Autodesk Inventor part; units mm, degrees
ref_plane "YZ Plane" through (0, 0, 0) normal (1, 0, 0) x (0, 1, 0)
ref_plane "XZ Plane" through (0, 0, 0) normal (0, 1, 0) x (-1, 0, 0)
ref_plane "XY Plane" through (0, 0, 0) normal (0, 0, 1) x (1, 0, 0)
sketch "Sketch1" plane through (0, 0, 0) normal (1, 0, 0) x (0, 1, 0)
  line L0 (-32.2, 0) -> (32.2, 0)
  line L1 (0, -4.2) -> (0, 4.2)
  circle A0 centre (-20, 0) radius 1.25
  circle A1 centre (-20, 0) radius 3
  circle A2 centre (20, 0) radius 3 construction
  line L2 (-20, 3) -> (20, 3)
  line L3 (-20, -3) -> (20, -3)
  line L4 (20, 3) -> (20, -3) construction
  line L5 (20, 2) -> (20, -2) construction
  arc A3 (20, -3) -> (20, 3) centre (20, 0) ccw
  circle A4 centre (-20, 0) radius 2.2678 construction
  circle A5 centre (20, 0) radius 1
  point P0 (0, 0)
  dimension "d4" = 6
  dimension "d7" = 40
  dimension "d8" = 2.5
  dimension "d10" = 0
  dimension "d30" = 2
extrude "ext_main" add sketch "Sketch1" along normal mid plane 3.5 contours A0 L0 A1 | L0 A1 A0 | A1 L2 L1 L0 | L0 L1 L3 A1 | L1 L2 A3 L0 A5 | L0 A5 A3 L3 L1
sketch "Sketch3" plane through (0, 0, 0) normal (1, 0, 0) x (0, 1, 0)
  arc A0 (-20, 3) -> (-20, -3) centre (-20, 0) ccw
  circle A1 centre (-20, 0) radius 1.25
  arc A2 (20, -3) -> (20, 3) centre (20, 0) ccw
  circle A3 centre (-20, 0) radius 3 construction
  circle A4 centre (20, 0) radius 3 construction
  line L0 (-17.7639, 2) -> (17.7639, 2) construction
  line L1 (-42.7, 0) -> (42.7, 0)
  line L2 (0, -4.2579) -> (0, 4.2579)
  line L3 (20, 3) -> (-20, 3)
  line L4 (16.6192, 2) -> (19.0141, 2.8334)
  arc A5 (20, 3) -> (19.0141, 2.8334) centre (20, 0) ccw
  line L5 (-16.8389, 2) -> (16.6192, 2)
  circle A6 centre (-20, 0) radius 2.75
  line L6 (-16.8389, 2) -> (-19.2882, 2.6563)
  arc A7 (19.0141, -2.8334) -> (20, -3) centre (20, 0) ccw
  line L7 (16.6192, -2) -> (-17.7639, -2) construction
  line L8 (-16.8389, -2) -> (-19.2882, -2.6563)
  line L9 (16.6192, -2) -> (-16.8389, -2)
  line L10 (16.6192, -2) -> (19.0141, -2.8334)
  point P0 (0, 0)
  dimension "d16" = 1
  dimension "d21" = 5.5
  dimension "d22" = 15
extrude "ext_cutaway" cut sketch "Sketch3" along normal through all both and the other way through all contours A6 L1 A1 | L1 A1 A6 | L5 L4 A5 A2 L1 L2 | L2 L1 A6 L6 L5 | A6 L1 L2 L9 L8 | L1 A2 A7 L10 L9 L2 keep common part
sketch "Sketch4" plane through (1.75, 0, 0) normal (1, 0, 0) x (0, 0, -1)
  arc A0 (2.8334, 19.0141) -> (-2.8334, 19.0141) centre (0, 20) ccw
  circle A1 centre (0, 20) radius 1
  circle A2 centre (0, 20) radius 3
  line L0 (-4.2, 0) -> (4.2, 0)
  line L1 (-3, 20) -> (3, 20) construction
  circle A3 centre (0, 20) radius 2 construction
  arc A4 (-1.4283, 21.4) -> (-1.4283, 18.6) centre (0, 20) ccw
  arc A5 (1.4283, 18.6) -> (1.4283, 21.4) centre (0, 20) ccw
  line L2 (-1.4283, 21.4) -> (1.4283, 21.4)
  line L3 (-1.4283, 18.6) -> (1.4283, 18.6)
  point P0 (0, 0)
  dimension "d23" = 4
  dimension "d25" = 2.8
extrude "ext_potshaft" add sketch "Sketch4" along normal blind 3.5 contours A2 A0
extrude "ext_cut_potshaft" cut sketch "Sketch4" against normal blind 1 contours L2 A5 L3 A4
equation "\"d8\" = screw_m2_bore_loose"
equation "\"d30\" = screw_m2_bore_selfthreading"
equation "\"d21\" = general_bore_smallersupport_diameter"
properties part number "empty"
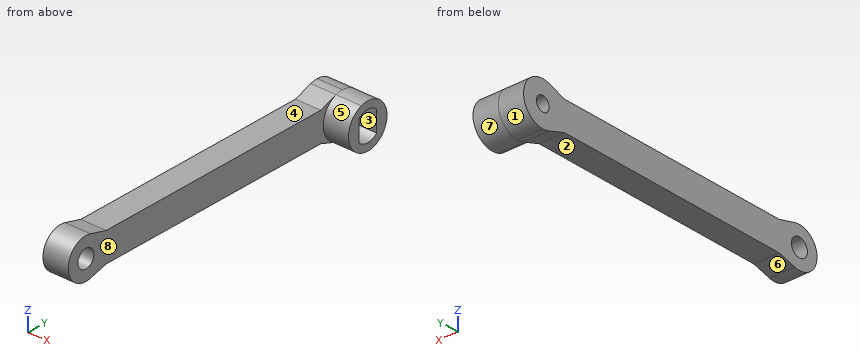
CAD build for the part. Positions are in the model's coordinates, mm. Face numbers are marked on the shaded views. A direction names the side the tool comes from. Coordinates: 2 decimals unless noted, no trailing zeros. Order: outer loops, then holes, each group sorted by start corner. A loop starts at its lowest first (then second) coordinate and runs counter-clockwise, first axis right, second up.
Item 1: Band-saw the part on D-D on y = -12. List the corners of the cut face in (x, z), plus the area to 3 significant figures.
Check sheet entries:
outline: (-1.75, -2) - (1.75, -2) - (1.75, 2) - (-1.75, 2) - close
area: 14.0 mm2
Item 2: Band-saw the part on B-B on y = -20. List the corners of the cut face in (x, z), plus the area to 3 significant figures.
Check sheet entries:
outline: (-1.75, -2.75) - (1.75, -2.75) - (1.75, -1.25) - (-1.75, -1.25) - close; (-1.75, 1.25) - (1.75, 1.25) - (1.75, 2.75) - (-1.75, 2.75) - close
area: 10.5 mm2
Item 3: Drill centre lines: L1, parallel to Z at x = 0.25, y = 20; L2, parallel to Z at x = -0.8, y = -20; L3, parallel to Y at x = 4.75, z = 0. Where is each one in solid material? Low to high.
Check sheet entries:
L1: z = -3 to -1, 1 to 3
L2: z = -2.75 to -1.25, 1.25 to 2.75
L3: y = 17 to 18.6, 21.4 to 23
Item 4: Pin check, flat tips, straight feed: pin 1 Ø1.2 at (y, z) = (20, 0) entering from -X; pin 2 Ø1 at (x, y) = (0, -16.5) entering from +Z; pin 3 Ø3 at (x, y) = (0.5, -3.5) entering from -Z; pin 4 Ø2 at (x, z) = (4, -0.5) entering from -Y. Stop position of each tip, or through.
Check sheet entries:
pin 1: passes through
pin 2: stops at z = 2.04
pin 3: stops at z = -2
pin 4: stops at y = 17
Item 5: Band-saw the part on C-C on x = 3.75. List the corners of the cut face in (y, z), plus the area to 3 significant figures.
Check sheet entries:
outline: circle Ø6 at (20, 0); hole (18.6, -1.43) arc R2 ccw to (21.4, -1.43) - (21.4, 1.43) arc R2 ccw to (18.6, 1.43) - close
area: 18.1 mm2
Item 6: Two-plate mould, pull along Y, no slides. Class the marked faces 6, 7 and 8: +Y half, -Y half, draft (parallel to the pull), parting line (faces both ways), or undercut.
Check sheet entries:
face 6: undercut
face 7: parting line
face 8: draft
Item 7: 3-axis set-ups, long thin cutter, end or side, ignore diameter. For the marked faces 1, 2, 3, 4 and 5: which of +Z, -Z, +X, -X, +Y, -Y reach the whole face in a straight line?
Check sheet entries:
face 1: +X, -X, +Y
face 2: -Z, +X, -X
face 3: +X
face 4: +Z, +X, -X
face 5: +X, -Y
Item 8: Band-saw the part on A-A on z = 0. List the corners of the cut face in (x, y), plus the area to 3 significant figures.
Check sheet entries:
outline: (-1.75, -22.75) - (1.75, -22.75) - (1.75, -21.25) - (-1.75, -21.25) - close; (-1.75, -18.75) - (1.75, -18.75) - (1.75, 17) - (5.25, 17) - (5.25, 18.6) - (0.75, 18.6) - (0.75, 19) - (-1.75, 19) - close; (-1.75, 21) - (0.75, 21) - (0.75, 21.4) - (5.25, 21.4) - (5.25, 23) - (-1.75, 23) - close
area: 155 mm2
